Job drawing, mm, ordinate dimensions from the low corner. One solid piece. Round coordinates to 2 decimals unless told otherwise and drop trailing zeros. Write each loop counter-clockwise with the first axis right and the second up, starting at its lowest first coordinate (ties: lowest second). Pieces come first, ordered by that corner, then holes.
1) Saw through at D-D (z = 12). Write the cut outline in (x, y).
2) Pull direction X, two halves, no side cores. Call the marked faces 1, 2 and 3: +X half, -X half, draft (parallel to the pull), parting line (faces both ways), or undercut.
3) Flat gauge pins, fed straight in: pin 1 (10 mm diameter, centred on y = 7.5, z = 56, fed in from +X); pin 2 (8 mm diameter, centred on y = 12, z = 77.5, fed in from -X); pin 3 (10 mm diameter, centred on x = 25, y = 2.5, fed in from +Z). Where does each tip first touch, or does it go through?
4) Saw through at B-B (y = 13.5). Write the cut outline in (x, z).
5) Wall check: probe 1 along Z at (x, y) = (68, 1) (1 decimal); probe 2 along Z at (x, y) = (62, 2.5) (1 decimal); probe 3 along X at (y, z) = (8, 52.5). Give the ranges that are in metal, low to high.
6) Saw through at A-A (x = 47.5). Write the cut outline in (y, z), plus the area to 3 significant figures.
7) Saw through at C-C (z = 68.5). Write the cut outline in (x, y) (1 decimal).
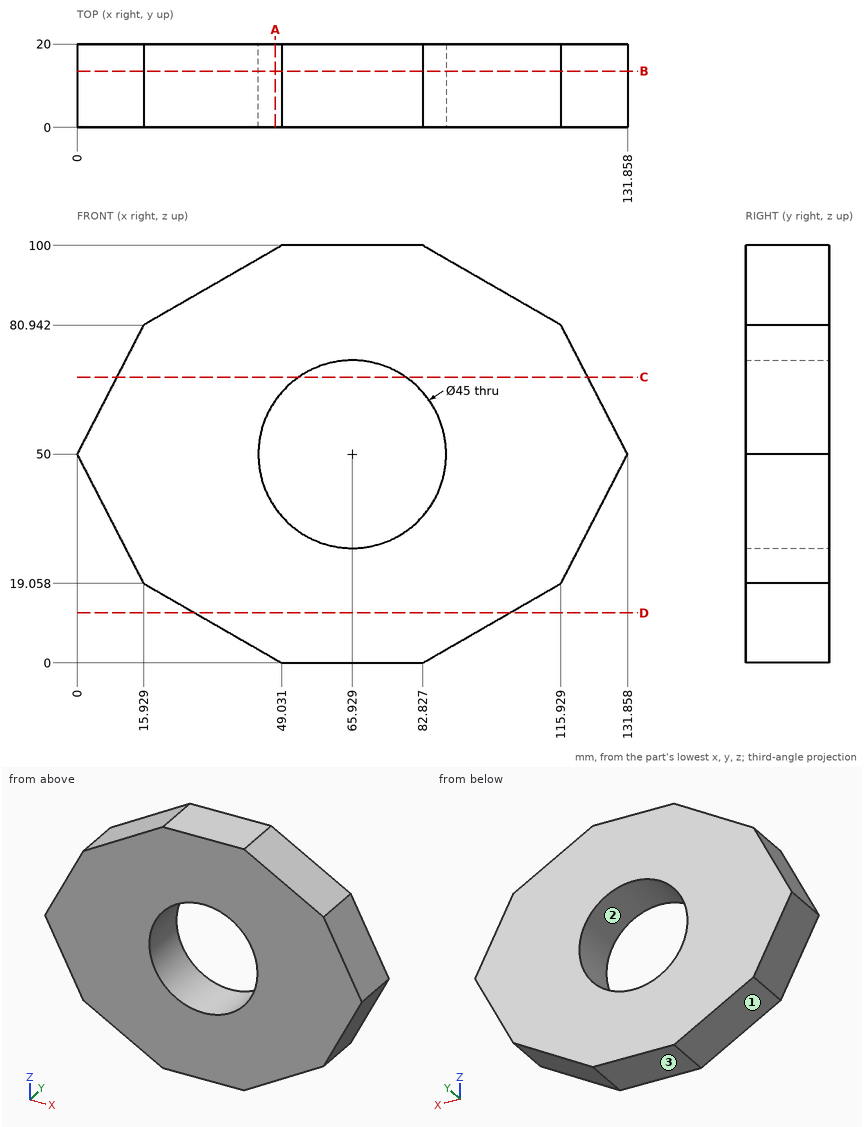
Evaluation:
1. outline: (28.19, 0) - (103.67, 0) - (103.67, 20) - (28.19, 20) - close
2. face 1: -X half
2. face 2: undercut
2. face 3: draft
3. pin 1: stops at x = 131.34
3. pin 2: stops at x = 12.1
3. pin 3: stops at z = 89.04
4. outline: (0, 50) - (15.93, 19.06) - (49.03, 0) - (82.83, 0) - (115.93, 19.06) - (131.86, 50) - (115.93, 80.94) - (82.83, 100) - (49.03, 100) - (15.93, 80.94) - close; hole circle Ø45 at (65.93, 50)
5. probe 1: z = 0 to 27.6, 72.4 to 100
5. probe 2: z = 0 to 27.8, 72.2 to 100
5. probe 3: x = 1.29 to 43.57, 88.29 to 130.57
6. outline: (0, 0.88) - (20, 0.88) - (20, 37.09) - (0, 37.09) - close; (0, 62.91) - (20, 62.91) - (20, 99.12) - (0, 99.12) - close
6. area: 1,450 mm2
7. outline: (9.5, 0) - (53.1, 0) - (53.1, 20) - (9.5, 20) - close; (78.7, 0) - (122.3, 0) - (122.3, 20) - (78.7, 20) - close
